Could you check a few things on this model? Use its own coordinates, in mm. A direction names the side the tool comes from. Coordinates: 2 decimals unless noted, no trailing zeros. Loops run counter-clockwise (first coordinate to the right, second up) from the corner with the lowest first, then second, coordinate; pieces in that order, holes last.
from build123d import *

# Parameters (mm, degrees)
SKETCH1_R               = 38.1127
BOSS_EXTRUDE1_DEPTH     = 9.525
SKETCH2_R               = 1.651
SKETCH2_R_2             = 11.8745
CUT_EXTRUDE1_DEPTH      = 10.525
SKETCH4_R               = 2.3749
CUT_EXTRUDE2_DEPTH      = 6.35
CIRPATTERN1_COUNT       = 3
SKETCH5_R               = 2.38125
CUT_EXTRUDE3_DEPTH      = 1.0000001
CUT_EXTRUDE3_DEPTH_BACK = 10.5250001


with BuildPart() as part:
    # Sketch1 → Boss-Extrude1 (new body)
    with BuildSketch(Plane(origin=(0, 0, 0), x_dir=(1, 0, 0), z_dir=(0, 1, 0))):
        Circle(SKETCH1_R)
    extrude(amount=BOSS_EXTRUDE1_DEPTH)

    # Sketch2 → Cut-Extrude1 (cut, through all)
    with BuildSketch(Plane(origin=(0, 9.525, 0), x_dir=(1, 0, 0), z_dir=(0, 1, 0))):
        with Locations((0, 29.464)):
            Circle(SKETCH2_R)
        with Locations((25.516572497, -14.732)):
            Circle(SKETCH2_R)
        with Locations((-25.516572497, -14.732)):
            Circle(SKETCH2_R)
        with Locations((-12.7, 10.16)):
            Circle(SKETCH2_R_2)
        with Locations((12.7, 10.16)):
            Circle(SKETCH2_R_2)
    extrude(amount=-CUT_EXTRUDE1_DEPTH, mode=Mode.SUBTRACT)

    # Sketch4 → Cut-Extrude2 (cut)
    with BuildSketch(Plane(origin=(19.05635, 0, -33.006566407), x_dir=(0, -1, 0), z_dir=(0.5, 0, -0.866025404))):
        with Locations((-4.7625, 0)):
            Circle(SKETCH4_R)
    cut_extrude2 = extrude(amount=-CUT_EXTRUDE2_DEPTH, mode=Mode.SUBTRACT)

    # CirPattern1: Cut-Extrude2 ×3 about axis
    cirpattern1_axis = Axis((0, 0, 0), (0, 1, 0))
    for i in range(1, CIRPATTERN1_COUNT):
        add(cut_extrude2.rotate(cirpattern1_axis, i * 360 / CIRPATTERN1_COUNT), mode=Mode.SUBTRACT)

    # Sketch5 → Cut-Extrude3 (cut, two sides)
    with BuildSketch(Plane(origin=(0, 9.525, 0), x_dir=(1, 0, 0), z_dir=(0, 1, 0))) as cut_extrude3_sk:
        with Locations((-15.875, -10.16)):
            Circle(SKETCH5_R)
        with Locations((15.875, -10.16)):
            Circle(SKETCH5_R)
    extrude(amount=CUT_EXTRUDE3_DEPTH, mode=Mode.SUBTRACT)
    extrude(cut_extrude3_sk.sketch, amount=-CUT_EXTRUDE3_DEPTH_BACK, mode=Mode.SUBTRACT)


solid = part.part
(1) Imagine slicing it at B-B, the plane x = -4.5. Write out the boundary of the cut face in (y, z) (3 decimals), and give its area (3 significant figures).
Answers:
outline: (0, -37.846) - (9.525, -37.846) - (9.525, -18.749) - (0, -18.749) - close; (0, -1.571) - (9.525, -1.571) - (9.525, 37.846) - (0, 37.846) - close
area: 557 mm2
(2) We'd pull the mould along Z, two halves only. Please class faces 1 (the face through (-30.245, 4.696, 23.191)), 2 (the face through (16.873, 2.497, -30.652)), 3 (the face through (-1, 0, -1)): +Z half, -Z half, draft (parallel to the pull), parting line (faces both ways), or undercut.
Answers:
face 1: parting line
face 2: undercut
face 3: draft
(3) Imagine slicing it at A-A, the plane z = -10.16. Write out the boundary of the cut face in (x, y) (1 decimal).
Answers:
outline: (-36.7, 0) - (-24.6, 0) - (-24.6, 9.5) - (-36.7, 9.5) - close; (-0.8, 0) - (0.8, 0) - (0.8, 9.5) - (-0.8, 9.5) - close; (24.6, 0) - (36.7, 0) - (36.7, 9.5) - (24.6, 9.5) - close
(4) Imagine slicing it at D-D, the plane x = -15.5. Write out the boundary of the cut face in (y, z) (1 decimal).
Answers:
outline: (0, -34.8) - (9.5, -34.8) - (9.5, -21.7) - (0, -21.7) - close; (0, 1.4) - (9.5, 1.4) - (9.5, 7.8) - (0, 7.8) - close; (0, 12.5) - (9.5, 12.5) - (9.5, 34.8) - (0, 34.8) - close
(5) Which directions (+Z, -Z, +X, -X, +Y, -Y) give clear straight access to the entire face, cutting with the end or side of a thin tool? Please do faces 4 (the face through (-31.763, 5, 0)), 5 (the face through (15.91, 4.8, 27.49)), 6 (the face through (10.126, 4.829, 1.432)).
Answers:
face 4: -X
face 5: none
face 6: +Y, -Y
(6) I need wall thicknesses on probe 1 along X at (y, z) = (6.75, 12); probe 2 along X at (y, z) = (7, -5); probe 3 along Z at (x, y) = (-14, 9.25). Which ranges of each line are inside material? Lowest first, please.
Answers:
probe 1: x = -36.17 to -17.39, -14.36 to 14.36, 17.39 to 36.17
probe 2: x = -37.78 to -23.39, -2.01 to 2.01, 23.39 to 37.78
probe 3: z = -35.45 to -21.96, 1.64 to 8.69, 11.63 to 35.45
(7) For pin 1 (4 mm diameter, centred on x = 19.5, y = 7, fed in from -Z); pin 2 (3 mm diameter, centred on x = 0, z = -29.464, fed in from -Y), each with a flat end and sliding along its axis, tell me the tip position at first contact or that it passes through.
Answers:
pin 1: stops at z = -33.86
pin 2: passes through
(8) Imagine slicing it at C-C, the plane y = 5.75. Write out the boundary of the cut face in (x, z) (1 decimal), and give its area (3 significant figures).
Answers:
outline: (-38.1, -2.2) arc R38.1 ccw to (17.2, -34) - (14, -28.6) - (17.8, -26.4) - (20.9, -31.9) arc R38.1 ccw to (20.9, 31.9) - (17.8, 26.4) - (14, 28.6) - (17.2, 34) arc R38.1 ccw to (-38.1, 2.2) - (-31.8, 2.2) - (-31.8, -2.2) - close; hole circle Ø3.3 at (-25.5, 14.7); hole circle Ø23.7 at (-12.7, -10.2); hole circle Ø4.8 at (-15.9, 10.2); hole circle Ø3.3 at (0, -29.5); hole circle Ø23.7 at (12.7, -10.2); hole circle Ø4.8 at (15.9, 10.2); hole circle Ø3.3 at (25.5, 14.7)
area: 3,530 mm2
